Autodesk Inventor part; units mm, degrees
ref_plane "Start Plane" through (0, 0, 0) normal (0, 0, 1) x (1, 0, 0)
ref_plane "End Plane" through (0, 0, 445.5965) normal (0, 0, 1) x (1, 0, 0)
ref_plane "YZ Plane" through (0, 0, 0) normal (1, 0, 0) x (0, 1, 0)
ref_plane "Start Plane" through (0, 0, 0) normal (0, 0, 1) x (1, 0, 0)
ref_plane "End Plane" through (0, 0, 445.5965) normal (0, 0, 1) x (1, 0, 0)
sketch "Sketch" plane through (0, 0, 0) normal (0, 0, 1) x (1, 0, 0)
  line L0 (-9.525, -8.0315) -> (-9.525, 8.0315)
  line L1 (-8.0315, 9.525) -> (8.0315, 9.525)
  line L2 (9.525, 8.0315) -> (9.525, -8.0315)
  line L3 (8.0315, -9.525) -> (-8.0315, -9.525)
  arc A0 (-9.525, -8.0315) -> (-8.0315, -9.525) centre (-8.0315, -8.0315) ccw
  arc A1 (-8.0315, 9.525) -> (-9.525, 8.0315) centre (-8.0315, 8.0315) ccw
  arc A2 (9.525, 8.0315) -> (8.0315, 9.525) centre (8.0315, 8.0315) ccw
  arc A3 (8.0315, -9.525) -> (9.525, -8.0315) centre (8.0315, -8.0315) ccw
  arc A4 (-8.0315, 8.2804) -> (-8.2804, 8.0315) centre (-8.0315, 8.0315) ccw
  line L4 (-8.0315, 8.2804) -> (8.0315, 8.2804)
  arc A5 (8.2804, 8.0315) -> (8.0315, 8.2804) centre (8.0315, 8.0315) ccw
  line L5 (8.2804, 8.0315) -> (8.2804, -8.0315)
  arc A6 (8.0315, -8.2804) -> (8.2804, -8.0315) centre (8.0315, -8.0315) ccw
  line L6 (8.0315, -8.2804) -> (-8.0315, -8.2804)
  arc A7 (-8.2804, -8.0315) -> (-8.0315, -8.2804) centre (-8.0315, -8.0315) ccw
  line L7 (-8.2804, -8.0315) -> (-8.2804, 8.0315)
  line L8 (0, 13.768) -> (0, -13.768) construction
  line L9 (-13.8012, 0) -> (13.9669, 0) construction
  dimension "d10" = 19.05
  dimension "d11" = 19.05
  dimension "d12" = 1.2446
  dimension "d15" = 9.525
  dimension "d16" = 9.525
  dimension "d17" = 1.4935
extrude "Body" add sketch "Sketch" along normal up to surface (445.5965 mm away) from surface at 0
sketch "Sketch3" plane through (0, 0, 0) normal (0, 0, 1) x (1, 0, 0)
  line L0 (0, 0) -> (10, 0)
ref_plane "Work Plane3" through (0, 0, 0) normal (0, -1, 0) x (1, 0, 0)
sketch "Sketch5" plane through (9.525, -8.0315, 445.5965) normal (1, 0, 0) x (0, 0, -1)
  line L0 (0, 16.063) -> (0, 0)
  line L1 (445.5965, 0) -> (0, 0)
  line L2 (445.5965, 16.063) -> (445.5965, 0)
  line L3 (445.5965, 16.063) -> (0, 16.063)
  circle A0 centre (206.1206, 8.0315) radius 4
  point P0 (445.5965, 8.0315)
  point P1 (445.5965, 8.0315)
  dimension "d20" = 8
extrude "Extrusion2" cut sketch "Sketch5" against normal through all contours A0
sketch "Sketch4" plane through (0, 0, 0) normal (0, -1, 0) x (1, 0, 0)
  line L0 (-2, 0) -> (12, 0)
  line L1 (-2, 445.5965) -> (12, 445.5965)
  dimension "d19" = 445.5965
equation "\"d10\" = G_H"
equation "\"d11\" = G_W"
equation "\"d12\" = G_T"
equation "\"d15\" = 0.5 * d10"
equation "\"d16\" = 0.5 * d11"
equation "\"d17\" = G_IR"
equation "\"d3\" = G_L"
equation "\"G_W\" = 19.05"
equation "\"G_H\" = 19.05"
equation "\"G_T\" = 1.2446"
equation "\"G_IR\" = 1.2 * G_T"
equation "\"G_L\" = d19"
equation "\"G_OFFSET_START\" = 0"
equation "\"G_OFFSET_END\" = 0"
equation "\"d14\" = G_OFFSET_END + B_L"
equation "\"B_L\" = 445.59646"
properties part number "ASTM A513 - 3/4 x 3/4 x 49/1000 - 17.543" material "Steel, Mild"
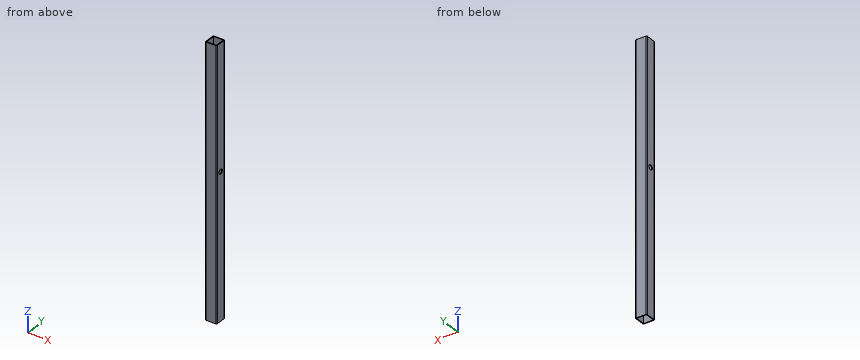
Could you check a few things on this model? Use its own coordinates, in mm. Round coordinates to 2 decimals unless told otherwise and drop trailing zeros. Loops run counter-clockwise (first coordinate to the right, second up) from the corner with the lowest first, then second, coordinate; pieces in that order, holes last. Notation, with made-up numbers: (27, 10) - (76, 10) arc R27 ccw to (76, 34) - close; hole circle Ø4 at (36.5, -11.5). An arc over 180 degrees is marked (long way). Answer in a Markdown table with one row per item. Add a question column.
(1) If we section it at B-B (y = 0): Please give me the cut outline in (x, z) (1 decimal).
(2) I need wall thicknesses on line 1 along Y through (x, z) = (2.25, 295) (3 decimals); line 2 along X through (y, z) = (8.5, 319). Which ranges of each line are inside material? Lowest first, please.
(3) If we section it at A-A (x = 2): Please give me the cut outline in (y, z) (1 decimal), plus the area to 3 significant figures.
Model answer:
| question | item | result |
|---|---|---|
| 1 | outline | (-9.5, 0) - (-8.3, 0) - (-8.3, 235.5) - (-9.5, 235.5) - close; (-9.5, 243.5) - (-8.3, 243.5) - (-8.3, 445.6) - (-9.5, 445.6) - close; (8.3, 0) - (9.5, 0) - (9.5, 235.5) - (8.3, 235.5) - close; (8.3, 243.5) - (9.5, 243.5) - (9.5, 445.6) - (8.3, 445.6) - close |
| 2 | line 1 | y = -9.525 to -8.28, 8.28 to 9.525 |
| 2 | line 2 | x = -9.45 to 9.45 |
| 3 | outline | (-9.5, 0) - (-8.3, 0) - (-8.3, 445.6) - (-9.5, 445.6) - close; (8.3, 0) - (9.5, 0) - (9.5, 445.6) - (8.3, 445.6) - close |
| 3 | area | 1,110 mm² |
